Geometry: see drawing. Coordinates: mm, zero at the bounding-box minimum. Coordinates: 2 decimals unless noted, no trailing zeros. Loops run counter-clockwise (first coordinate to the right, second up) from the corner with the lowest first, then second, coordinate; pieces in that order, holes last. Notation, with made-up numbers: (-38.5, 36.25) -> (10.5, 36.25) arc R21 cw to (10.5, 55.25) -> close; hole circle Ø9 at (42.25, 57.5). An arc over 180 degrees is marked (long way). One line per question, with ' | ' between items. Start each with the question number.
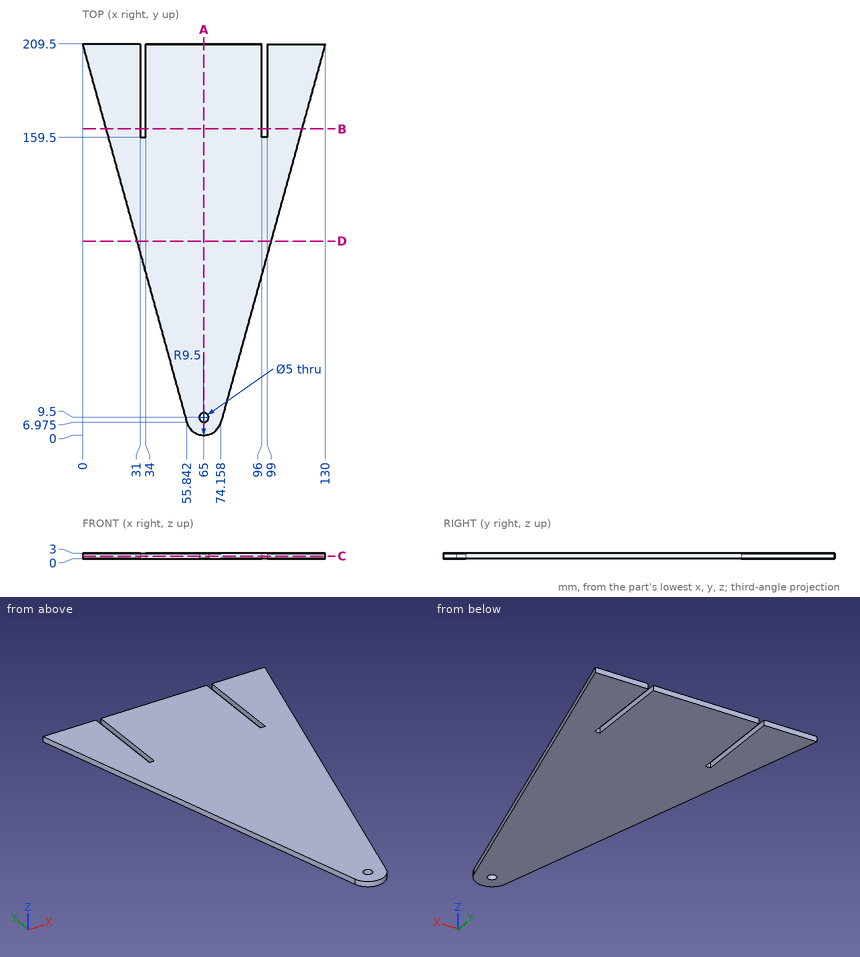
(1) Cut plane A-A, the plane x = 65. Return the cut outline in (y, z).
(2) Contact query for flat-ended pins moving along their axis: pin 1 Ø1.5 at (x, y) = (37, 128) entering from -Z; pin 2 Ø1.5 at (y, z) = (190.5, 1.5) entering from -X; pin 3 Ø0.9 at (x, z) = (33, 2) entering from +Y. Output: stop coordinate, or through.
(3) Cut plane D-D, the plane y = 104. Return the cut outline in (x, z).
(4) Cut plane C-C, the plane z = 1.5. Return the cut outline in (x, y) (1 decimal).
(5) Cut plane B-B, the plane y = 164. Return the cut outline in (x, z), and give its area (3 significant figures).
(6) Ray query, L1, parallel to X at y = 160.5, z = 2.6; L2, parallel to Y at x = 65, z = 1.1; L3, parallel to X at y = 197.5, z = 2.45. Return the intervals inside material, ascending.
Here are the results:
1) outline: (0, 0) -> (7, 0) -> (7, 3) -> (0, 3) -> close; (12, 0) -> (209.5, 0) -> (209.5, 3) -> (12, 3) -> close
2) pin 1: stops at z = 0 | pin 2: stops at x = 5.03 | pin 3: stops at y = 159.5
3) outline: (29.09, 0) -> (100.91, 0) -> (100.91, 3) -> (29.09, 3) -> close
4) outline: (0, 209.5) -> (55.8, 7) arc R9.5 ccw to (74.2, 7) -> (130, 209.5) -> (99, 209.5) -> (99, 159.5) -> (96, 159.5) -> (96, 209.5) -> (34, 209.5) -> (34, 159.5) -> (31, 159.5) -> (31, 209.5) -> close; hole circle Ø5 at (65, 9.5)
5) outline: (12.55, 0) -> (31, 0) -> (31, 3) -> (12.55, 3) -> close; (34, 0) -> (96, 0) -> (96, 3) -> (34, 3) -> close; (99, 0) -> (117.45, 0) -> (117.45, 3) -> (99, 3) -> close | area: 297 mm2
6) L1: x = 13.51 to 31, 34 to 96, 99 to 116.49 | L2: y = 0 to 7, 12 to 209.5 | L3: x = 3.31 to 31, 34 to 96, 99 to 126.69
